Check sheet for the drawn part. Datum: minimum x, y, z corner. Units: mm. A direction names the side the tool comes from. Round coordinates to 2 decimals unless told otherwise and drop trailing zeros. Loops run counter-clockwise (first coordinate to the right, second up) from the corner with the lowest first, then second, coordinate; pieces in that order, holes last. Notation, with made-up numbers: (37.5, 67) - (70.5, 67) arc R18 cw to (70.5, 83) - close; hole circle Ø6 at (18, 4). An arc over 180 degrees is marked (long way). Use CSV: the item, a comma, the result in double quotes.
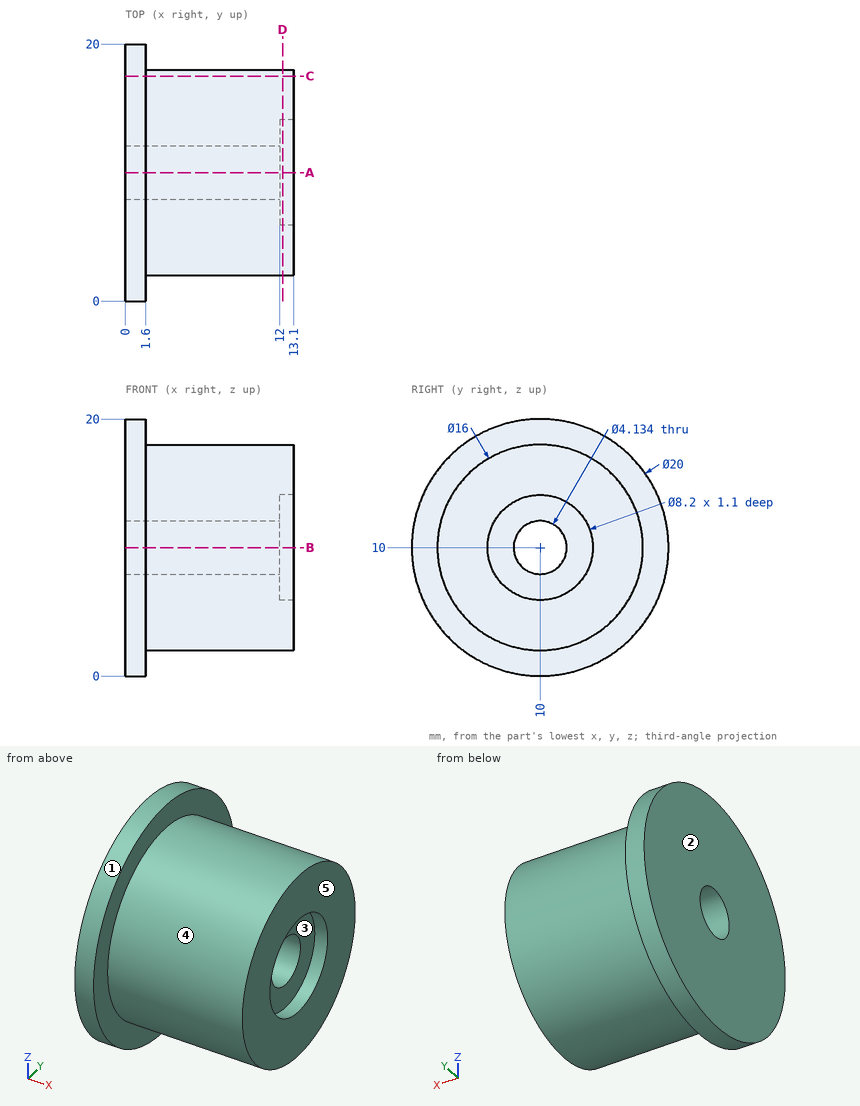
1) Thickness scan on probe 1 along Z at (x, y) = (7.25, 10); probe 2 along Z at (x, y) = (12.8, 10); probe 3 along X at (y, z) = (16.5, 17.5). Record the ranges inside material, lowest first. Write a range as [from, to].
Returned:
probe 1,"z = [2, 7.93], [12.07, 18]"
probe 2,"z = [2, 5.9], [14.1, 18]"
probe 3,"x = [0, 1.6]"
2) Cross-section at C-C, the plane y = 17.5. Record the cut outline in (x, z).
Returned:
outline,"(0, 3.39) - (1.6, 3.39) - (1.6, 7.22) - (13.1, 7.22) - (13.1, 12.78) - (1.6, 12.78) - (1.6, 16.61) - (0, 16.61) - close"
3) Mould release check, pull along Y, two halves, no side actions. Record for the marked faces 1, 2 and 3: +Y half, -Y half, draft (parallel to the pull), parting line (faces both ways), or undercut.
Returned:
face 1,"parting line"
face 2,"draft"
face 3,"undercut"
4) Cross-section at A-A, the plane y = 10. Record the cut outline in (x, z).
Returned:
outline,"(0, 0) - (1.6, 0) - (1.6, 2) - (13.1, 2) - (13.1, 5.9) - (12, 5.9) - (12, 7.93) - (0, 7.93) - close; (0, 12.07) - (12, 12.07) - (12, 14.1) - (13.1, 14.1) - (13.1, 18) - (1.6, 18) - (1.6, 20) - (0, 20) - close"
5) Cross-section at D-D, the plane x = 12.25. Record the cut outline in (y, z), then the cut area to 3 significant figures.
Returned:
outline,"circle Ø16 at (10, 10); hole circle Ø8.2 at (10, 10)"
area,"148 mm²"
6) Access from +Z, -Z, +X, -X, +Y, -Y to the whole of each face (thin tool, end or side, straight path). Record for the marked faces 4 and 5.
Returned:
face 4,"+X"
face 5,"+Z, -Z, +X, +Y, -Y"
7) Gauge pin test, flat ends, axial feed: pin 1 Ø4 at (x, y) = (11, 18) entering from +Z; pin 2 Ø6.5 at (y, z) = (9.5, 10.5) entering from +X; pin 3 Ø4 at (x, y) = (10.5, 17) entering from +Z (3 decimals). Record the tip position at first contact, or that the pin passes through.
Returned:
pin 1,"stops at z = 15.29"
pin 2,"stops at x = 12"
pin 3,"stops at z = 16.245"
